Answer from the drawing. Dimensions are ordinates in mm from the lowest x, y and z of the part. Give positions to 0.01 mm unless a question says otherwise; leave off trailing zeros. Order: outer loops, then holes, each group sorted by start corner. A loop starts at its lowest first (then second) coordinate and runs counter-clockwise, first axis right, second up.
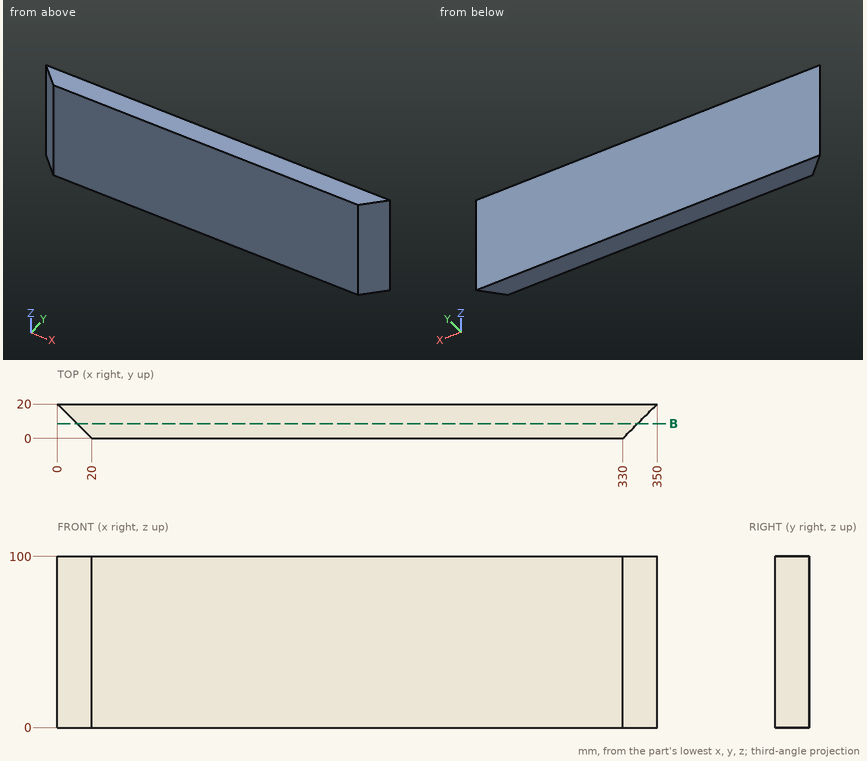
1) Given pin 1 (12 mm diameter, centred on y = 6.5, z = 52, fed in from -X); pin 2 (1 mm diameter, centred on y = 4.5, z = 29.5, fed in from -X); pin 3 (1 mm diameter, centred on y = 16.5, z = 78, fed in from +X), each flat-ended and moving along its own axis, determine where each tip first touches the part or whether it passes through.
Final values:
pin 1: stops at x = 7.5
pin 2: stops at x = 15
pin 3: stops at x = 347
2) The part is cut by section B-B on y = 8.5. Determine the outline of the cut face in (x, z), and give its area (3 significant figures).
Final values:
outline: (11.5, 0) - (338.5, 0) - (338.5, 100) - (11.5, 100) - close
area: 32,700 mm2
3) Consider L1, parallel to X at y = 1.5, z = 5; L2, parallel to X at y = 2.5, z = 87.5. Determine where each line is inside the solid, lowest interval first.
Final values:
L1: x = 18.5 to 331.5
L2: x = 17.5 to 332.5
